Here's how the part is built. I have some questions about the finished solid (model axes, mm). A direction names the side the tool comes from. Round coordinates to 2 decimals unless told otherwise and drop trailing zeros. Order: outer loops, then holes, each group sorted by start corner. A loop starts at its lowest first (then second) coordinate and runs counter-clockwise, first axis right, second up. Notation, with made-up numbers: (-23.5, 4) -> (2.5, 4) arc R12 cw to (2.5, 23) -> close; hole circle Ø8 at (-18.75, 14). An arc over 180 degrees is marked (long way). One line per item, written item: value.
```python
from build123d import *

# Parameters (mm, degrees)
SKETCH1_W           = 28.6
SKETCH1_H           = 5
BOSS_EXTRUDE1_DEPTH = 0.25
SKETCH2_W           = 5
SKETCH2_H           = 11
BOSS_EXTRUDE2_DEPTH = 0.25
BOSS_EXTRUDE3_DEPTH = 0.25
FILLET3_R           = 2
FILLET4_R           = 2
SKETCH4_W           = 6.639451807
SKETCH4_H           = 5
CUT_EXTRUDE1_DEPTH  = 1.5
SKETCH5_W           = 5
SKETCH5_H           = 3.595357205
BOSS_EXTRUDE4_DEPTH = 0.25
FILLET5_R           = 2
FILLET6_R           = 2
BOSS_EXTRUDE5_DEPTH = 0.25
CUT_EXTRUDE2_DEPTH  = 0.25
SKETCH8_W           = 6.875858175
SKETCH8_H           = 9.336027613
CUT_EXTRUDE3_DEPTH  = 5.25


with BuildPart() as part:
    # Sketch1 → Boss-Extrude1 (new body)
    with BuildSketch(Plane(origin=(0, 0, 0), x_dir=(1, 0, 0), z_dir=(0, 1, 0))):
        with Locations((-2.737209302, 3.434883721)):
            Rectangle(SKETCH1_W, SKETCH1_H)
    extrude(amount=BOSS_EXTRUDE1_DEPTH)

    # Sketch2 → Boss-Extrude2 (add)
    with BuildSketch(Plane.ZY.offset(17.037209302)):
        with Locations((-3.434883721, 5.75)):
            Rectangle(SKETCH2_W, SKETCH2_H)
    extrude(amount=-BOSS_EXTRUDE2_DEPTH)

    # Sketch3 → Boss-Extrude3 (add)
    with BuildSketch(Plane(origin=(11.562790698, 0, 0), x_dir=(0, 0, -1), z_dir=(1, 0, 0))):
        Polygon((0.934883721, 0.25), (5.936255285, 0.25), (5.936255285, 2.75), (4.435569503, 4.205909665), (4.435569503, 5.205909665), (3.435569503, 5.205909665), (2.435569503, 5.205909665), (2.435569503, 4.205909665), (0.934883721, 2.75), align=None)
    extrude(amount=-BOSS_EXTRUDE3_DEPTH)

    # Fillet3
    fillet3_edges = [part.edges().sort_by_distance(p)[0] for p in [
        (-16.787209302, 0.25, -3.434883721),
        (11.312790698, 0.25, -3.434883721),
    ]]
    fillet(fillet3_edges, radius=FILLET3_R)

    # Fillet4
    # the kernel refuses this fillet: 2 mm, written as the material it takes off along each edge
    with BuildSketch(Plane(origin=(11.562790698, 0, -10.934883721), x_dir=(-1, 0, 0), z_dir=(0, 0, 1))) as fillet4_piece_1:
        with BuildLine():
            CenterArc((FILLET4_R, -FILLET4_R), FILLET4_R, 90, 90)
            Line((0, -FILLET4_R), (0, 0))
            Line((0, 0), (FILLET4_R, 0))
        make_face()
    extrude(amount=15, mode=Mode.SUBTRACT)
    with BuildSketch(Plane(origin=(-17.037209302, 0, 4.065116279), x_dir=(0, 1, 0), z_dir=(0, 0, -1))) as fillet4_piece_2:
        with BuildLine():
            CenterArc((FILLET4_R, FILLET4_R), FILLET4_R, 180, 90)
            Line((0, FILLET4_R), (0, 0))
            Line((0, 0), (FILLET4_R, 0))
        make_face()
    extrude(amount=15, mode=Mode.SUBTRACT)

    # Sketch4 → Cut-Extrude1 (cut)
    with BuildSketch(Plane.XZ):
        with Locations((6.243064795, -3.434883721)):
            Rectangle(SKETCH4_W, SKETCH4_H)
    extrude(amount=-CUT_EXTRUDE1_DEPTH, mode=Mode.SUBTRACT)


with BuildPart() as cut_extrude1_piece_1:
    # of the separate pieces the step leaves, piece 1, a body of its own (cut_extrude1_pieces)
    add(part.part.solids().sort_by_distance((-16.787209302, 2.25, -5.934883721))[0])

    # Sketch5 → Boss-Extrude4 (add)
    with BuildSketch(Plane(origin=(2.923338891, 0, 0), x_dir=(0, 0, -1), z_dir=(1, 0, 0))):
        with Locations((3.434883721, 1.797678603)):
            Rectangle(SKETCH5_W, SKETCH5_H)
    extrude(amount=BOSS_EXTRUDE4_DEPTH)

    # Fillet5
    fillet5_edges = [cut_extrude1_piece_1.edges().sort_by_distance(p)[0] for p in [
        (2.923338891, 0.25, -3.434883721),
    ]]
    fillet(fillet5_edges, radius=FILLET5_R)

    # Fillet6
    fillet6_edges = [cut_extrude1_piece_1.edges().sort_by_distance(p)[0] for p in [
        (3.173338891, 0, -3.434883721),
    ]]
    fillet(fillet6_edges, radius=FILLET6_R)

    # Sketch6 → Boss-Extrude5 (add)
    with BuildSketch(Plane(origin=(3.173338891, 0, 0), x_dir=(0, 0, -1), z_dir=(1, 0, 0))):
        Polygon((0.934883721, 2.75), (2.435569503, 4.205909665), (2.435569503, 5.205909665), (4.435569503, 5.205909665), (4.435569503, 4.205909665), (5.934883721, 2.75), align=None)
    extrude(amount=-BOSS_EXTRUDE5_DEPTH)

    # Sketch7 → Cut-Extrude2 (cut)
    with BuildSketch(Plane(origin=(3.173338891, 0, 0), x_dir=(0, 0, -1), z_dir=(1, 0, 0))):
        Polygon((1.806239664, 3.595357205), (0.934883721, 3.595357205), (0.934883721, 2.797678603), align=None)
        Polygon((5.064324161, 3.595357205), (5.934883721, 3.595357205), (5.934883721, 2.797678603), align=None)
    extrude(amount=-CUT_EXTRUDE2_DEPTH, mode=Mode.SUBTRACT)


with BuildPart() as cut_extrude1_piece_2:
    # of the separate pieces the step leaves, piece 2, a body of its own (cut_extrude1_pieces)
    add(part.part.solids().sort_by_distance((9.562790698, 0, -5.934883721))[0])

    # Sketch8 → Cut-Extrude3 (cut)
    with BuildSketch(Plane(origin=(0, 0, -5.936255285), x_dir=(-1, 0, 0), z_dir=(0, 0, -1))):
        with Locations((-11.197633492, 2.582921844)):
            Rectangle(SKETCH8_W, SKETCH8_H)
    extrude(amount=-CUT_EXTRUDE3_DEPTH, mode=Mode.SUBTRACT)


solid = cut_extrude1_piece_1.part
```
Q1. For P1, Ø2.5, axis at x = -8.5, z = -3, coming from the +Y side; P2, Ø3, axis at x = -14, z = -3, coming from the +Y side; P3, Ø1, axis at y = 10, z = -5.5, coming from the +X side; P4, Ø5, axis at x = -13, y = 3.5, coming from the +Z side, each with a flat end and sliding along its axis, tell me the tip position at first contact or that it passes through.
Answers:
P1: y = 0.25
P2: y = 0.38
P3: x = -16.79
P4: through
Q2. If we mould it in two halves opening along X, with no side actions, what happens to faces 3 (the face through (-7, 0.25, -3)), 4 (the face through (-16.217, 0.851, -3.4)), 5 (the face through (2.6, 0.6, -3.5)), 6 (the face through (-7, 0, -3))? For each: pulls with the +X half, pulls with the -X half, needs draft (parallel to the pull), parting line crosses it, or undercut.
Answers:
face 3: undercut
face 4: undercut
face 5: pulls with the +X half
face 6: needs draft
Q3. I want a section at B-B on z = -3.1. Write out the boundary of the cut face in (x, y).
Answers:
outline: (-17.04, 2) arc R2 ccw to (-15.04, 0) -> (1.17, 0) arc R2 ccw to (3.17, 2) -> (3.17, 5.21) -> (2.92, 5.21) -> (2.92, 2.25) arc R2 cw to (0.92, 0.25) -> (-14.79, 0.25) arc R2 cw to (-16.79, 2.25) -> (-16.79, 11.25) -> (-17.04, 11.25) -> close
Q4. I want a section at A-A on y = 5. Write out the boundary of the cut face in (x, z), then the cut area to 3 significant figures.
Answers:
outline: (-17.04, -5.93) -> (-16.79, -5.93) -> (-16.79, -0.93) -> (-17.04, -0.93) -> close; (2.92, -4.44) -> (3.17, -4.44) -> (3.17, -2.44) -> (2.92, -2.44) -> close
area: 1.75 mm2
Q5. I want a section at C-C on x = -6.5. Write out the boundary of the cut face in (y, z).
Answers:
outline: (0, -5.93) -> (0.25, -5.93) -> (0.25, -0.93) -> (0, -0.93) -> close
Q6. I want a section at D-D on y = 3. Write out the boundary of the cut face in (x, z).
Answers:
outline: (-17.04, -5.93) -> (-16.79, -5.93) -> (-16.79, -0.93) -> (-17.04, -0.93) -> close; (2.92, -5.71) -> (3.17, -5.71) -> (3.17, -1.16) -> (2.92, -1.16) -> close
Q7. Which directions (+Z, -Z, +X, -X, +Y, -Y) give clear straight access to the entire face, cutting with the end or side of a thin tool? Please do faces 1 (the face through (-16.787, 7, -3)), 2 (the face through (3.173, 3, -3)).
Answers:
face 1: +Z, -Z, +Y
face 2: +Z, -Z, +X, +Y, -Y
Q8. I need wall thicknesses on line 1 along X through (y, z) = (2.25, -4.2); line 2 along Y through (x, z) = (-9, -3.1); line 3 along X through (y, z) = (6, -4.75). Which ranges of each line are inside material? Lowest first, please.
Answers:
line 1: -17.04 to -16.79, 2.92 to 3.17
line 2: 0 to 0.25
line 3: -17.04 to -16.79
